Here's how the part is built. I have some questions about the finished solid (model axes, mm). A direction names the side the tool comes from. Give positions to 0.01 mm unless a question says otherwise; leave off trailing zeros. Loops run counter-clockwise (first coordinate to the right, second up) from the corner with the lowest first, then second, coordinate; pieces in that order, holes last. Notation, with made-up numbers: M 17,30.5 L 64,30.5 A33 ccw 64,62.5 Z; hole C 0.5,81.25 d6. An arc over 180 degrees is marked long. Answer as CSV lines item,"result". Start each with the question number.
Item 1: For faces 1 (the flat face through (1, -18, 2.875)), 2 (the cylindrical face through (-17.655, -59.976, 12.903)), which set-ups out of +Z, -Z, +X, -X, +Y, -Y let a thin tool reach every point of the face, with its end or its side?
Item 2: Will these pins go through, and if not, where does the flat tip stop? P1, Ø1, axis at x = -2.5, z = 6.5, coming from the -Y side; P2, Ø5, axis at x = 0, z = 11, coming from the -Y side; P3, Ø2, axis at x = -2, y = -31, coming from the -Z side; P4, Ø8, axis at x = -15.5, z = 10, coming from the +Y side.
Item 3: I want a section at A-A on z = 11.75. List the corners of the cut face in (x, y) for me.
Item 4: I want a section at B-B on x = -7. List the corners of the cut face in (y, z) for me, plus the area to 3 significant figures.
Item 5: I want a section at D-D on z = 5. List the corners of the cut face in (x, y) for me, plus the area to 3 significant figures.
Item 6: If I drill on line 1 along Y through (x, z) = (-14.75, 16.25); line 2 along Y through (x, z) = (0.5, 5.5); line 3 along X through (y, z) = (-43.5, 15.75), over which ranges is the centre line in solid material (lowest first)? Write a range as from..to.
Item 7: I want a section at C-C on z = 15.75. List the corners of the cut face in (x, y) for me.
from build123d import *

# Parameters (mm, degrees)
BOSS_EXTRUDE1_DEPTH = 2
SKETCH1_3_R         = 1
BOSS_EXTRUDE2_DEPTH = 4
SKETCH1_4_R         = 1
BOSS_EXTRUDE3_DEPTH = 12


with BuildPart() as part:
    # Sketch1 → Boss-Extrude1 (new body)
    with BuildSketch(Plane.XY.offset(14.87534902)):
        with BuildLine():
            Line((2.748026099, -19.086356488), (-15.614663255, -59.821649221))
            ThreePointArc((-15.614663255, -59.821649221), (-18.259886239, -60.823045928), (-19.261282946, -58.177822944))
            Line((-19.261282946, -58.177822944), (-0.898593592, -17.442530211))
            ThreePointArc((-0.898593592, -17.442530211), (1.746629392, -16.441133504), (2.748026099, -19.086356488))
        make_face()
    extrude(amount=BOSS_EXTRUDE1_DEPTH)

    # Sketch1<3> → Boss-Extrude2 (add)
    with BuildSketch(Plane.XY.offset(14.87534902)):
        with Locations((-17.4379731, -58.999736083)):
            Circle(SKETCH1_3_R)
    extrude(amount=-BOSS_EXTRUDE2_DEPTH)

    # Sketch1<4> → Boss-Extrude3 (add)
    with BuildSketch(Plane.XY.offset(14.87534902)):
        with Locations((0.924716254, -18.26444335)):
            Circle(SKETCH1_4_R)
    extrude(amount=-BOSS_EXTRUDE3_DEPTH)


solid = part.part
Result:
1,face 1,"-Z, +X, -X, +Y, -Y"
1,face 2,"-Z"
2,P1,"through"
2,P2,"y = -19.26"
2,P3,"z = 14.88"
2,P4,"y = -58"
3,outline,"C -17.44,-59 d2; C 0.92,-18.26 d2"
4,outline,"M -40.71,14.88 L -30.98,14.88 L -30.98,16.88 L -40.71,16.88 Z"
4,area,"19.5 mm^2"
5,outline,"C 0.92,-18.26 d2"
5,area,"3.14 mm^2"
6,line 1,"-57.9..-48.17"
6,line 2,"-19.17..-17.36"
6,line 3,"-12.64..-8.26"
7,outline,"M -19.26,-58.18 A2 ccw -15.61,-59.82 L 2.75,-19.09 A2 ccw -0.9,-17.44 Z"
